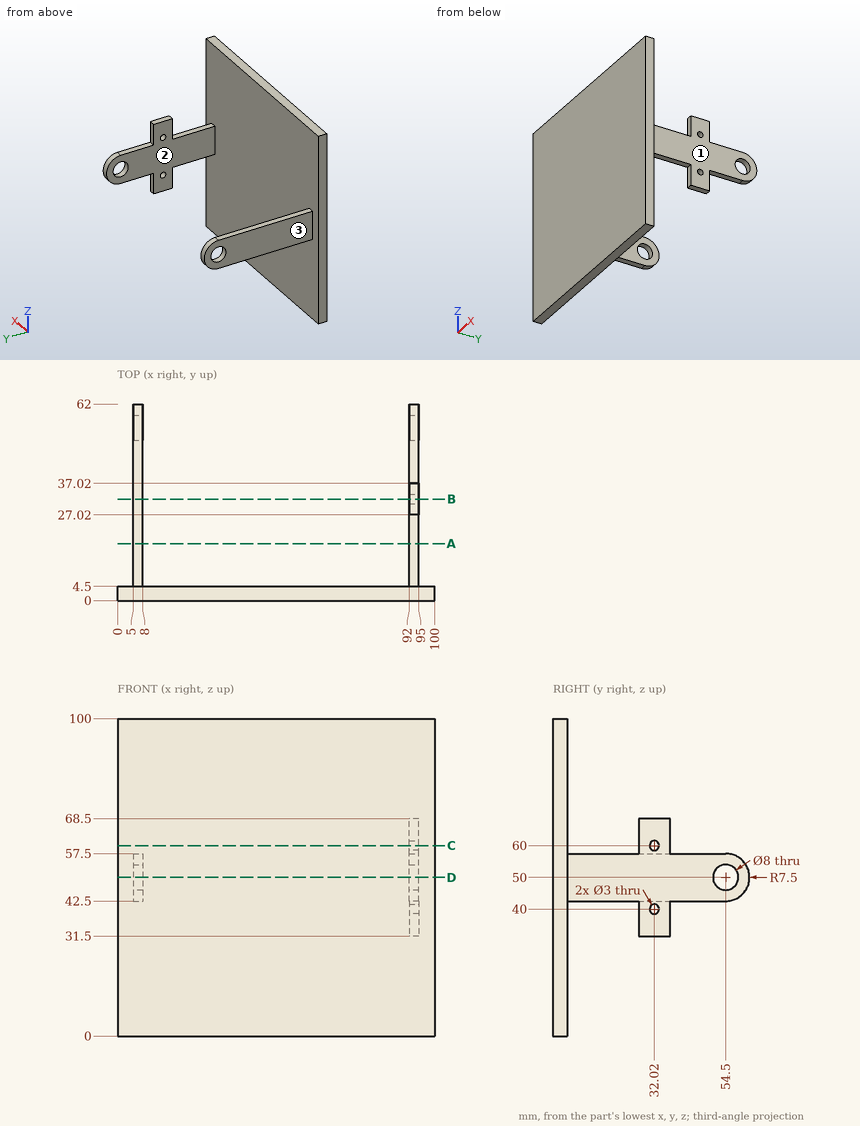
Print and shaded views of the part. All mm, measured from the part's lowest x, y and z. A direction names the side the tool comes from. Give positions to 0.01 mm unless a question says otherwise; leave off trailing zeros. Write each loop counter-clockwise with the first axis right and the second up, starting at its lowest first coordinate (ties: lowest second). Pieces come first, ordered by that corner, then holes. Notation, with made-up numbers: M 62.5,39 L 86.5,39 A13 cw 86.5,49 Z; hole C 83,54 d4. An arc over 180 degrees is marked long. Use a Markdown table: item, result.
1) Pin check, flat tips, straight feed: pin 1 (3.5 mm diameter, centred on y = 32.02, z = 40, fed in from +X); pin 2 (1.5 mm diameter, centred on x = 93.5, y = 30.5, fed in from -Z); pin 3 (2.5 mm diameter, centred on x = 93.5, y = 44, fed in from -Z); pin 4 (6.5 mm diameter, centred on y = 54.5, z = 50, fed in from -X). Stop position of each tip, or through.
Responses:
| item | result |
|---|---|
| pin 1 | stops at x = 95 |
| pin 2 | stops at z = 31.5 |
| pin 3 | stops at z = 42.5 |
| pin 4 | passes through |
2) Cut at B-B (y = 32.02). List the corners of the cut face in (x, z), and give its area (3 significant figures).
Responses:
| item | result |
|---|---|
| outline | M 5,42.5 L 8,42.5 L 8,57.5 L 5,57.5 Z; M 92,31.5 L 95,31.5 L 95,38.5 L 92,38.5 Z; M 92,41.5 L 95,41.5 L 95,58.5 L 92,58.5 Z; M 92,61.5 L 95,61.5 L 95,68.5 L 92,68.5 Z |
| area | 138 mm2 |
3) Tool access for the marked faces 1, 2 and 3: list every direction of +Z, -Z, +X, -X, +Y, -Y with a clear straight run to the whole face (end or side of a thin tool).
Responses:
| item | result |
|---|---|
| face 1 | +Z, -Z, +X, +Y |
| face 2 | +Z, -Z, +Y |
| face 3 | +Z, -Z, -X, +Y |
4) Drill centre lines: line 1 (Y direction, x = 93.25, z = 40); line 2 (Y direction, x = 6.4, z = 50); line 3 (X direction, y = 26, z = 47.5). Where is each one in solid material? Low to high. Write a range as from..to.
Responses:
| item | result |
|---|---|
| line 1 | y = 0..4.5, 27.02..30.52, 33.52..37.02 |
| line 2 | y = 0..50.5, 58.5..62 |
| line 3 | x = 5..8, 92..95 |
5) Cut at A-A (y = 18). List the corners of the cut face in (x, z).
Responses:
| item | result |
|---|---|
| outline | M 5,42.5 L 8,42.5 L 8,57.5 L 5,57.5 Z; M 92,42.5 L 95,42.5 L 95,57.5 L 92,57.5 Z |
6) Cut at D-D (z = 50). List the corners of the cut face in (x, y).
Responses:
| item | result |
|---|---|
| outline | M 0,0 L 100,0 L 100,4.5 L 95,4.5 L 95,50.5 L 92,50.5 L 92,4.5 L 8,4.5 L 8,50.5 L 5,50.5 L 5,4.5 L 0,4.5 Z; M 5,58.5 L 8,58.5 L 8,62 L 5,62 Z; M 92,58.5 L 95,58.5 L 95,62 L 92,62 Z |
7) Cut at C-C (z = 60). List the corners of the cut face in (x, y), and give its area (3 significant figures).
Responses:
| item | result |
|---|---|
| outline | M 0,0 L 100,0 L 100,4.5 L 0,4.5 Z; M 92,27.02 L 95,27.02 L 95,30.52 L 92,30.52 Z; M 92,33.52 L 95,33.52 L 95,37.02 L 92,37.02 Z |
| area | 471 mm2 |
